Autodesk Fusion 360 part; units mm, degrees
sketch "Sketch2" plane through (0, 0, 0) normal (0, 0, 1) x (1, 0, 0)
  line L0 (0, 0) -> (76, 0)
  line L1 (76, 0) -> (76, 70)
  line L2 (76, 70) -> (0, 70)
  line L3 (0, 70) -> (0, 0)
  dimension "d20" = 76
  dimension "d21" = 70
extrude "Extrude1" add sketch "Sketch2" along normal blind 2.9
sketch "Sketch3" plane through (0, 0, 2.9) normal (0, 0, 1) x (-1, 0, 0)
  line L0 (0, -70) -> (0, 0)
  line L1 (0, 0) -> (-76, 0)
  line L2 (-76, 0) -> (-76, -70)
  line L3 (-76, -70) -> (0, -70)
  line L4 (0, -70) -> (-7, -70)
  line L5 (-7, -70) -> (-7, -69)
  line L6 (-7, -69) -> (-14, -69)
  line L7 (-14, -69) -> (-14, -67)
  line L8 (-14, -67) -> (-9, -67)
  line L9 (-9, -67) -> (-9, -62)
  line L10 (-9, -62) -> (-7, -62)
  line L11 (-7, -62) -> (-7, -69)
  line L12 (-9, -67) -> (-68, -67)
  line L13 (-68, -67) -> (-63, -67)
  line L14 (-63, -67) -> (-63, -69)
  line L15 (-63, -69) -> (-70, -69)
  line L16 (-70, -69) -> (-70, -62)
  line L17 (-70, -62) -> (-68, -62)
  line L18 (-68, -62) -> (-68, -67)
  line L19 (-68, -67) -> (-68, -3)
  line L20 (-68, -3) -> (-63, -3)
  line L21 (-63, -3) -> (-63, -1)
  line L22 (-63, -1) -> (-70, -1)
  line L23 (-70, -1) -> (-70, -8)
  line L24 (-70, -8) -> (-68, -8)
  line L25 (-68, -3) -> (-68, -8)
  line L26 (-9, -67) -> (-9, -3)
  line L27 (-9, -3) -> (-14, -3)
  line L28 (-14, -3) -> (-14, -1)
  line L29 (-14, -1) -> (-7, -1)
  line L30 (-7, -1) -> (-7, -8)
  line L31 (-7, -8) -> (-9, -8)
  line L32 (-9, -3) -> (-9, -8)
  dimension "d24" = 7
  dimension "d25" = 1
  dimension "d26" = 7
  dimension "d27" = 2
  dimension "d28" = 5
  dimension "d29" = 5
  dimension "d30" = 2
  dimension "d31" = 59
  dimension "d32" = 5
  dimension "d33" = 2
  dimension "d34" = 64
  dimension "d35" = 5
  dimension "d36" = 2
  dimension "d37" = 7
  dimension "d38" = 7
  dimension "d39" = 2
  dimension "d40" = 64
  dimension "d41" = 5
  dimension "d42" = 2
  dimension "d43" = 7
  dimension "d44" = 7
extrude "Extrude2" add sketch "Sketch3" along normal blind 5 contours L19 L20 L21 L22 L23 L24 L25 | L12 L13 L14 L15 L16 L17 L18 L19 | L26 L27 L28 L29 L30 L31 L32 | L6 L7 L8 L9 L10 L11 L12 L26
extrude "Extrude3" cut 1 faces at (25.3333, 46.6667, 0) along direction (0, 0, 1) blind 1
sketch "Sketch4" plane through (0, 0, 2.9) normal (0, 0, 1) x (-1, 0, 0)
  line L0 (-14, -3) -> (-14, -1)
  line L1 (-14, -1) -> (-7, -1)
  line L2 (-7, -1) -> (-7, -8)
  line L3 (-7, -8) -> (-9, -8)
  line L4 (-9, -8) -> (-9, -3)
  line L5 (-9, -3) -> (-14, -3)
  line L6 (-9, -67) -> (-9, -62)
  line L7 (-9, -62) -> (-7, -62)
  line L8 (-7, -62) -> (-7, -69)
  line L9 (-7, -69) -> (-14, -69)
  line L10 (-14, -69) -> (-14, -67)
  line L11 (-14, -67) -> (-9, -67)
  line L12 (-63, -3) -> (-68, -3)
  line L13 (-68, -3) -> (-68, -8)
  line L14 (-68, -8) -> (-70, -8)
  line L15 (-70, -8) -> (-70, -1)
  line L16 (-70, -1) -> (-63, -1)
  line L17 (-63, -1) -> (-63, -3)
  line L18 (-63, -67) -> (-63, -69)
  line L19 (-63, -69) -> (-70, -69)
  line L20 (-70, -69) -> (-70, -62)
  line L21 (-70, -62) -> (-68, -62)
  line L22 (-68, -62) -> (-68, -67)
  line L23 (-68, -67) -> (-63, -67)
  line L24 (0, -70) -> (0, 0)
  line L25 (0, 0) -> (-76, 0)
  line L26 (-76, 0) -> (-76, -70)
  line L27 (-76, -70) -> (0, -70)
  line L28 (0, -70) -> (-4, -70)
  line L29 (-4, -70) -> (-6, -70)
  line L30 (-6, -70) -> (-6, -50)
  line L31 (-6, -50) -> (-4, -50)
  line L32 (-4, -50) -> (-4, -70)
  line L33 (-76, -70) -> (-72.5, -70)
  line L34 (-72.5, -70) -> (-71, -70)
  line L35 (-71, -70) -> (-71, -50)
  line L36 (-71, -50) -> (-72.5, -50)
  line L37 (-72.5, -50) -> (-72.5, -70)
  line L38 (0, -70) -> (0, -35)
  line L39 (0, -35) -> (-68, -35)
  line L40 (-4, -20) -> (-4, 0)
  line L41 (-4, 0) -> (-6, 0)
  line L42 (-6, 0) -> (-6, -20)
  line L43 (-6, -20) -> (-4, -20)
  line L44 (-71, 0) -> (-71, -20)
  line L45 (-72.5, 0) -> (-71, 0)
  line L46 (-72.5, -20) -> (-72.5, 0)
  line L47 (-71, -20) -> (-72.5, -20)
  dimension "d49" = 4
  dimension "d50" = 2
  dimension "d51" = 20
  dimension "d52" = 3.5
  dimension "d53" = 20
  dimension "d54" = 35
extrude "Extrude4" add sketch "Sketch4" along normal blind 3 contours L27 L29 L30 L31 L32 | L25 L40 L41 L42 L43 | L27 L34 L35 L36 L37 | L25 L44 L45 L46 L47
sketch "Sketch5" plane through (0, 0, 1) normal (0, 0, -1) x (1, 0, 0)
  line L0 (0, 0) -> (0, -70)
  line L1 (0, -70) -> (76, -70)
  line L2 (76, -70) -> (76, 0)
  line L3 (76, 0) -> (0, 0)
  line L4 (0, 0) -> (76, 0)
  line L5 (76, 0) -> (76, -70)
  line L6 (76, -70) -> (0, -70)
  line L7 (0, -70) -> (0, 0)
extrude "Extrude5" add sketch "Sketch5" along normal blind 0.6
equation "d54 = ( 70 / 2 ) * 1 mm"
Read the model definition and answer for the solid it produces. Units are mm, in the model's axes. A direction names the side the tool comes from. Give positions to 0.01 mm unless a question says otherwise; leave off trailing zeros. Order: outer loops, then holes, each group sorted by start corner. A loop starts at its lowest first (then second) coordinate and runs counter-clockwise, first axis right, second up. Notation, with made-up numbers: (58.5, 62) -> (98.5, 62) arc R26 cw to (98.5, 100) -> close; hole circle Ø7 at (41, 16). An arc over 180 degrees is marked (long way). Write item = value, one per line.
1. A cutting plane is placed at B-B, the plane x = 5. Write down the section's boundary in (y, z), and give its area (3 significant figures).
Numbers:
outline = (0, 0.4) -> (70, 0.4) -> (70, 5.9) -> (50, 5.9) -> (50, 2.9) -> (20, 2.9) -> (20, 5.9) -> (0, 5.9) -> close
area = 295 mm²
2. The mould has two halves that part along Y. Classify faces 5 (the face through (11, 3, 5)), 6 (the face through (8, 4, 7.9)), 7 (the face through (10, 69, 5)), 8 (the face through (68, 6, 5)): +Y half, -Y half, draft (parallel to the pull), parting line (faces both ways), or undercut.
Numbers:
face_5 = undercut
face_6 = draft
face_7 = +Y half
face_8 = undercut
3. A cutting plane is placed at C-C, the plane z = 4.5. Count the separate pieces of the cut face and the enclosed holes in it, and give its area (3 significant figures).
Numbers:
separate_pieces = 8
enclosed_holes = 0
area = 236 mm²
4. Straight lines are drawn through the part: line 1 along X through (y, z) = (6, 5.5); line 2 along Y through (x, z) = (72, 5.75); line 3 along X through (y, z) = (58, 5.75). For each, find the intervals that lie inside material, in ascending order.
Numbers:
line_1 = 4 to 6, 7 to 9, 68 to 70, 71 to 72.5
line_2 = 0 to 20, 50 to 70
line_3 = 4 to 6, 71 to 72.5
5. A cutting plane is placed at A-A, the plane y = 17.5. Write down the section's boundary in (x, z), and give its area (4 significant figures).
Numbers:
outline = (0, 0.4) -> (76, 0.4) -> (76, 2.9) -> (72.5, 2.9) -> (72.5, 5.9) -> (71, 5.9) -> (71, 2.9) -> (6, 2.9) -> (6, 5.9) -> (4, 5.9) -> (4, 2.9) -> (0, 2.9) -> close
area = 200.5 mm²
6. For faces 1 (the face through (65, 67, 5)), 2 (the face through (67, 2, 7.9)), 3 (the face through (14, 68, 5)), 4 (the face through (5, 50, 4)), determine the directions among +Z, -Z, +X, -X, +Y, -Y from which every point of the face is accessible in a straight line to the end or side of a thin tool.
Numbers:
face_1 = +Z
face_2 = +Z, +X, -X, +Y, -Y
face_3 = +Z, +Y, -Y
face_4 = +Z, +X, -X
7. Given pin 1 (4 mm diameter, centred on y = 65.5, z = 5.5, fed in from -X); pin 2 (0.6 mm diameter, centred on x = 5, y = 60, fed in from +Z); pin 3 (3 mm diameter, centred on x = 10.5, y = 53, fed in from +Z), each flat-ended and moving along its own axis, determine where each tip first touches the part or whether it passes through.
Numbers:
pin_1 = 4
pin_2 = 5.9
pin_3 = 2.9
8. A cutting plane is placed at D-D, the plane y = 30. Write down the section's boundary in (x, z), and give its area (3 significant figures).
Numbers:
outline = (0, 0.4) -> (76, 0.4) -> (76, 2.9) -> (0, 2.9) -> close
area = 190 mm²
